from build123d import *

# Parameters (mm, degrees)
SKETCH3_R                = 13.5382
SKETCH3_R_2              = 10.5156
BOSS_EXTRUDE1_DEPTH      = 0.6223
BOSS_EXTRUDE1_DEPTH_BACK = 0.6223
CUT_EXTRUDE1_DEPTH       = 14.5382


with BuildPart() as part:
    # Sketch3 → Boss-Extrude1 (new body, two sides)
    with BuildSketch(Plane(origin=(0, 0, 0), x_dir=(1, 0, 0), z_dir=(0, 1, 0))) as boss_extrude1_sk:
        Circle(SKETCH3_R)
        Circle(SKETCH3_R_2, mode=Mode.SUBTRACT)
    extrude(amount=BOSS_EXTRUDE1_DEPTH)
    extrude(boss_extrude1_sk.sketch, amount=-BOSS_EXTRUDE1_DEPTH_BACK)

    # Sketch4 → Cut-Extrude1 (cut, through all)
    with BuildSketch(Plane.XY):
        Polygon((2.838309027, 1.280985718), (-2.9315561, -1.050191113), (-2.838309027, -1.280985718), (2.9315561, 1.050191113), align=None)
    extrude(amount=CUT_EXTRUDE1_DEPTH, mode=Mode.SUBTRACT)


solid = part.part
The listing builds one solid part. Answer for the finished solid, in the listing's coordinates (mm). A direction names the side the tool comes from. Give positions to 0.01 mm unless a question says otherwise; leave off trailing zeros. Order: outer loops, then holes, each group sorted by start corner. A loop starts at its lowest first (then second) coordinate and runs counter-clockwise, first axis right, second up. Notation, with made-up numbers: (55, -3) - (90, -3) arc R12 cw to (90, 17) - close; hole circle Ø6 at (33, 49.5). An arc over 180 degrees is marked (long way). Use one line per item in the form item = value.
1) Find section D-D on y = 0.25. Determine the outline of the cut face in (x, z).
Verdict:
outline = (0.29, 10.51) - (0.29, 13.54) arc R13.54 ccw (long way) to (0.95, 13.5) - (0.95, 10.47) arc R10.52 cw (long way) to start
2) This flat-tipped pin is pushed along its axis until it touches: pin 1 (5 mm diameter, centred on x = -7.5, z = -5.5, fed in from -Y). Where does it stop, or does it pass through?
Verdict:
pin_1 = -0.62
3) Find section A-A on z = 4.75. Determine the outline of the cut face in (x, y).
Verdict:
outline = (-12.68, -0.62) - (-9.38, -0.62) - (-9.38, 0.62) - (-12.68, 0.62) - close; (9.38, -0.62) - (12.68, -0.62) - (12.68, 0.62) - (9.38, 0.62) - close
4) The mould has two halves that part along X. Classify faces 1 (the flat face through (0.31, -0.01, 11.92)), 2 (the flat face through (-8.1, -0.622, 7)): released by +X, released by -X, zero draft, split by the parting line, or undercut.
Verdict:
face_1 = undercut
face_2 = zero draft
5) For faces 3 (the flat face through (-8.1, 0.622, 7)), 4 (the flat face through (-0.31, 0.01, 11.92)), determine the directions among +Z, -Z, +X, -X, +Y, -Y from which every point of the face is accessible in a straight line to the end or side of a thin tool.
Verdict:
face_3 = +Z, -Z, +X, -X, +Y
face_4 = +Z
6) Consider probe 1 along Z at (x, y) = (0, 0.25); probe 2 along X at (y, z) = (-0.5, -2.75). Determine where each line is inside the solid, lowest interval first. Write a range as [from, to].
Verdict:
probe_1 = [-13.54, -10.52], [10.52, 13.54]
probe_2 = [-13.26, -10.15], [10.15, 13.26]
7) Find section C-C on x = 0. Determine the outline of the cut face in (y, z), and give its area (3 significant figures).
Verdict:
outline = (-0.62, -13.54) - (0.62, -13.54) - (0.62, -10.52) - (-0.62, -10.52) - close; (-0.62, 10.52) - (-0.13, 10.52) - (-0.13, 13.54) - (-0.62, 13.54) - close; (0.13, 10.52) - (0.62, 10.52) - (0.62, 13.54) - (0.13, 13.54) - close
area = 6.71 mm^2
8) Find section B-B on x = -8.25. Determine the outline of the cut face in (y, z), and give its area (3 significant figures).
Verdict:
outline = (-0.62, -10.73) - (0.62, -10.73) - (0.62, -6.52) - (-0.62, -6.52) - close; (-0.62, 6.52) - (0.62, 6.52) - (0.62, 10.73) - (-0.62, 10.73) - close
area = 10.5 mm^2
